from build123d import *

# Parameters (mm, degrees)
F3_DEPTH      = 55.6485557387
F3_DEPTH_BACK = 55.6485557387
F5_DEPTH      = 55.6485557387
F5_DEPTH_BACK = 55.6485557387


with BuildPart() as f1:
    # F0 (on Front) → F1 (revolve)
    with BuildSketch(Plane.XZ):
        with BuildLine():
            ThreePointArc((-55.6475557387, 0), (0, -55.6475557387), (55.6475557387, 0))
            Line((55.6475557387, 0), (-55.6475557387, 0))
        make_face()
    revolve(axis=Axis((0, 0, 0), (1, 0, 0)))

    # F2 (on Front) → F3 (cut, two sides)
    with BuildSketch(Plane.XZ) as f3_sk:
        Polygon((58.5763789713, 38.7402810156), (10.7213417068, 0), (70.8241611719, -11.8484022096), align=None)
    extrude(amount=-F3_DEPTH, mode=Mode.SUBTRACT)
    extrude(f3_sk.sketch, amount=F3_DEPTH_BACK, mode=Mode.SUBTRACT)

    # F4 (on Top) → F5 (cut, two sides)
    with BuildSketch(Plane.XY) as f5_sk:
        Polygon((71.6229304671, 0), (-63.6352449656, 0), (-62.3039603233, -69.3597495556), (71.6229304671, -69.3597495556), align=None)
    extrude(amount=-F5_DEPTH, mode=Mode.SUBTRACT)
    extrude(f5_sk.sketch, amount=F5_DEPTH_BACK, mode=Mode.SUBTRACT)


solid = f1.part
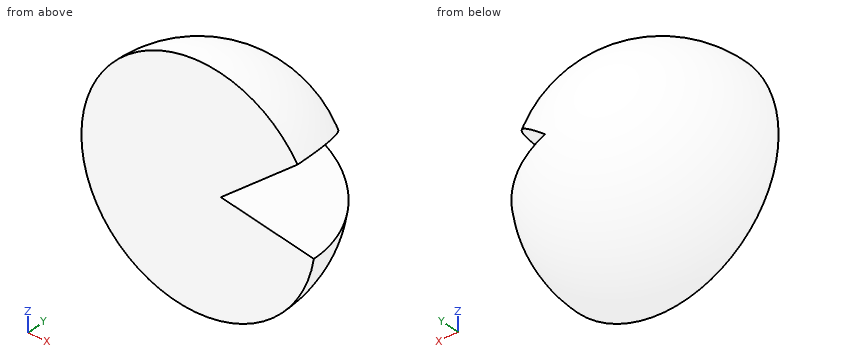
Input: part model. Units: mm. Frame: model coordinates. Round coordinates to 2 decimals unless told otherwise and drop trailing zeros. Loops run counter-clockwise (first coordinate to the right, second up) from the corner with the lowest first, then second, coordinate; pieces in that order, holes last. Notation, with made-up numbers: (-21.75, -31) -> (-9.75, -31) arc R12 ccw to (-9.75, -18) -> close; hole circle Ø5 at (-15.5, -24). An arc over 180 degrees is marked (long way). Answer as a JSON object with one key per item and string values. Group by question number.
1) Pin query (flat end, axial travel): pin 1 (3 mm diameter, centred on y = 7.5, z = -17, fed in from +X); pin 2 (10 mm diameter, centred on x = -27.5, z = -34, fed in from +Y); pin 3 (2 mm diameter, centred on x = 24, z = 20, fed in from +Y). Return the tip coordinate at first contact, or that it passes through.
2) Section query A-A on x = 14.5. Output: boundary loops of the cut face in (y, z).
3) Section query D-D on x = -25. Output: boundary loops of the cut face in (y, z), plus the area to 3 significant figures.
4) Section query B-B on y = 15.5. Output: boundary loops of the cut face in (x, z), plus the area to 3 significant figures.
5) Section query C-C on z = 36.5. Output: boundary loops of the cut face in (x, y), plus the area to 3 significant figures.
6) Ray query, L1, parallel to X at y = 3, z = -17.5; L2, parallel to Z at x = 20.5, y = 41; L3, parallel to Y at x = 5, z = -29. Return the intervals inside material, ascending.
Reply:
{
 "1": {"pin 1": "stops at x = 52.96", "pin 2": "stops at y = 39.96", "pin 3": "stops at y = 46.71"},
 "2": {"outline": "(0, -53.73) arc R53.73 ccw to (53.72, -0.74) -> (0, -0.74) -> close; (0, 3.06) -> (53.64, 3.06) arc R53.73 ccw to (0, 53.73) -> close"},
 "3": {"outline": "(0, -49.72) arc R49.72 ccw to (0, 49.72) -> close", "area": "3,880 mm2"},
 "4": {"outline": "(10.72, 0) -> (45.45, 28.12) arc R53.45 ccw (long way) to (52.8, -8.29) -> close", "area": "8,160 mm2"},
 "5": {"outline": "(-42, 0) -> (42, 0) arc R42 ccw to start", "area": "2,770 mm2"},
 "6": {"L1": "x = -52.74 to 52.74", "L2": "z = -31.55 to -1.93, 7.92 to 31.55", "L3": "y = 0 to 47.23"}
}
